Work out the finished part from the listing and answer in its coordinate system (mm). Face numbers are marked on the shaded views. A direction names the side the tool comes from. Coordinates: 2 decimals unless noted, no trailing zeros. Write each loop counter-clockwise with the first axis right and the second up, starting at its lowest first coordinate (ties: lowest second). Pieces come first, ordered by that corner, then holes. Notation, with made-up numbers: M 77.25,28.25 L 118.25,28.25 A23 cw 118.25,50.25 Z; hole C 12.5,3.5 d2. An arc over 180 degrees is marked long. Answer as CSV lines item,"result". Start each with the question number.
(1) For the marked faces 1 and 2, determine the directions among +Z, -Z, +X, -X, +Y, -Y from which every point of the face is accessible in a straight line to the end or side of a thin tool.
(2) Find the intervals of material crossed by L1, parallel to X at y = 1.75, z = 23.5; L2, parallel to Z at x = 3, y = 9.5; L3, parallel to X at y = 14, z = -27, in increasing order. Write a range as [from, to].
(3) A cutting plane is placed at C-C on x = 29. Give the vertices of the cut face in (y, z).
(4) A cutting plane is placed at A-A on y = 10.5. Give the vertices of the cut face in (x, z).
(5) The mould has two halves that part along X. Classify the marked faces 3, 4 and 5: released by +X, released by -X, zero draft, split by the parting line, or undercut.
(6) A cutting plane is placed at D-D on y = 5.25. Give the vertices of the cut face in (x, z).
(7) A flat-ended cylindrical pin translates along its axis: P1, Ø14, axis at x = 10, z = -7.5, coming from the +Y side. Find the tip coordinate at first contact, or state that the pin passes through.
(8) A cutting plane is placed at B-B on z = 1. Give the vertices of the cut face in (x, y).
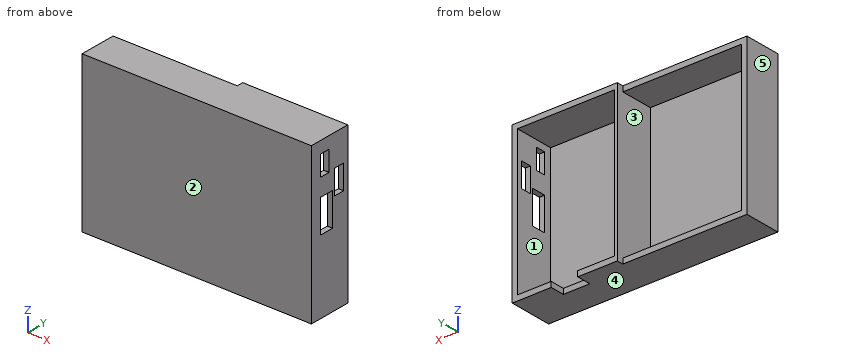
from build123d import *

# Parameters (mm, degrees)
BOSS_EXTRUDE1_DEPTH = 12.5
BOSS_EXTRUDE2_DEPTH = 15
SKETCH1_7_W         = 1
SKETCH1_7_H         = 55
BOSS_EXTRUDE3_DEPTH = 15
SKETCH1_10_W        = 45
SKETCH1_10_H        = 55
SKETCH1_10_W_2      = 36.8
SKETCH1_10_W_3      = 1
BOSS_EXTRUDE5_DEPTH = 1.5
SKETCH2_W           = 7.6828
SKETCH2_H           = 3.785279572
SKETCH2_W_2         = 12.5
SKETCH2_H_2         = 5.4
SKETCH2_W_3         = 9.2
SKETCH2_H_3         = 4.03174267
CUT_EXTRUDE1_DEPTH  = 10
SKETCH3_W           = 10
SKETCH3_H           = 5.5
CUT_EXTRUDE2_DEPTH  = 10


with BuildPart() as part:
    # Sketch1 → Boss-Extrude1 (new body)
    with BuildSketch(Plane(origin=(0, 0, 0), x_dir=(1, 0, 0), z_dir=(0, 1, 0))):
        Polygon((22.5, -27.5), (22.5, -29.5), (-24.5, -29.5), (-24.5, 29.5), (22.5, 29.5), (22.5, 27.5), (-22.5, 27.5), (-22.5, -27.5), align=None)
    extrude(amount=BOSS_EXTRUDE1_DEPTH)

    # Sketch1_5 → Boss-Extrude2 (add)
    with BuildSketch(Plane(origin=(0, 0, 0), x_dir=(1, 0, 0), z_dir=(0, 1, 0))):
        Polygon((22.5, -27.5), (23.5, -27.5), (60.3, -27.5), (60.3, 27.5), (23.5, 27.5), (22.5, 27.5), (22.5, 29.5), (23.5, 29.5), (62.3, 29.5), (62.3, -29.5), (23.5, -29.5), (22.5, -29.5), align=None)
    extrude(amount=BOSS_EXTRUDE2_DEPTH)

    # Sketch1_7 → Boss-Extrude3 (add)
    with BuildSketch(Plane(origin=(0, 0, 0), x_dir=(1, 0, 0), z_dir=(0, 1, 0))):
        with Locations((23, 0)):
            Rectangle(SKETCH1_7_W, SKETCH1_7_H)
    extrude(amount=BOSS_EXTRUDE3_DEPTH)

    # Sketch1_10 → Boss-Extrude5 (add)
    with BuildSketch(Plane(origin=(0, 0, 0), x_dir=(1, 0, 0), z_dir=(0, 1, 0))):
        Polygon((22.5, -27.5), (22.5, -29.5), (-24.5, -29.5), (-24.5, 29.5), (22.5, 29.5), (22.5, 27.5), (-22.5, 27.5), (-22.5, -27.5), align=None)
        Rectangle(SKETCH1_10_W, SKETCH1_10_H)
        with Locations((41.9, 0)):
            Rectangle(SKETCH1_10_W_2, SKETCH1_10_H)
        with Locations((23, 0)):
            Rectangle(SKETCH1_10_W_3, SKETCH1_10_H)
        Polygon((22.5, -27.5), (23.5, -27.5), (60.3, -27.5), (60.3, 27.5), (23.5, 27.5), (22.5, 27.5), (22.5, 29.5), (23.5, 29.5), (62.3, 29.5), (62.3, -29.5), (23.5, -29.5), (22.5, -29.5), align=None)
    extrude(amount=-BOSS_EXTRUDE5_DEPTH)

    # Sketch2 → Cut-Extrude1 (cut)
    with BuildSketch(Plane(origin=(62.3, 0, 0), x_dir=(0, 0, -1), z_dir=(1, 0, 0))):
        with Locations((-21.1586, 4.57741645)):
            Rectangle(SKETCH2_W, SKETCH2_H)
        with Locations((-4.4202, 5.380056236)):
            Rectangle(SKETCH2_W_2, SKETCH2_H_2)
        with Locations((-13.060208334, 11.084128665)):
            Rectangle(SKETCH2_W_3, SKETCH2_H_3)
    extrude(amount=-CUT_EXTRUDE1_DEPTH, mode=Mode.SUBTRACT)

    # Sketch3 → Cut-Extrude2 (cut)
    with BuildSketch(Plane(origin=(0, 0, -29.5), x_dir=(-1, 0, 0), z_dir=(0, 0, -1))):
        with Locations((-42.5, 12.25)):
            Rectangle(SKETCH3_W, SKETCH3_H)
    extrude(amount=-CUT_EXTRUDE2_DEPTH, mode=Mode.SUBTRACT)


solid = part.part
Here are the results:
1,face 1,"+Y"
1,face 2,"+Z, -Z, +X, -X, -Y"
2,L1,"x = [-24.5, -22.5], [22.5, 23.5], [60.3, 62.3]"
2,L2,"z = [-29.5, -27.5], [27.5, 29.5]"
2,L3,"x = [22.5, 23.5], [60.3, 62.3]"
3,outline,"M -1.5,-29.5 L 15,-29.5 L 15,-27.5 L 0,-27.5 L 0,27.5 L 15,27.5 L 15,29.5 L -1.5,29.5 Z"
4,outline,"M -24.5,-29.5 L 37.5,-29.5 L 37.5,-27.5 L 23.5,-27.5 L 23.5,27.5 L 60.3,27.5 L 60.3,17.66 L 62.3,17.66 L 62.3,29.5 L -24.5,29.5 Z; M 47.5,-29.5 L 62.3,-29.5 L 62.3,8.46 L 60.3,8.46 L 60.3,-27.5 L 47.5,-27.5 Z; hole M -22.5,-27.5 L 22.5,-27.5 L 22.5,27.5 L -22.5,27.5 Z"
5,face 3,"undercut"
5,face 4,"zero draft"
5,face 5,"released by -X"
6,outline,"M -24.5,-29.5 L 62.3,-29.5 L 62.3,-1.83 L 60.3,-1.83 L 60.3,-27.5 L 23.5,-27.5 L 23.5,27.5 L 60.3,27.5 L 60.3,25 L 62.3,25 L 62.3,29.5 L -24.5,29.5 Z; M 60.3,10.67 L 62.3,10.67 L 62.3,17.32 L 60.3,17.32 Z; hole M -22.5,-27.5 L 22.5,-27.5 L 22.5,27.5 L -22.5,27.5 Z"
7,P1,"stops at y = 0"
8,outline,"M -24.5,-1.5 L 62.3,-1.5 L 62.3,2.68 L 60.3,2.68 L 60.3,0 L 23.5,0 L 23.5,15 L 22.5,15 L 22.5,0 L -22.5,0 L -22.5,12.5 L -24.5,12.5 Z; M 60.3,8.08 L 62.3,8.08 L 62.3,15 L 60.3,15 Z"
